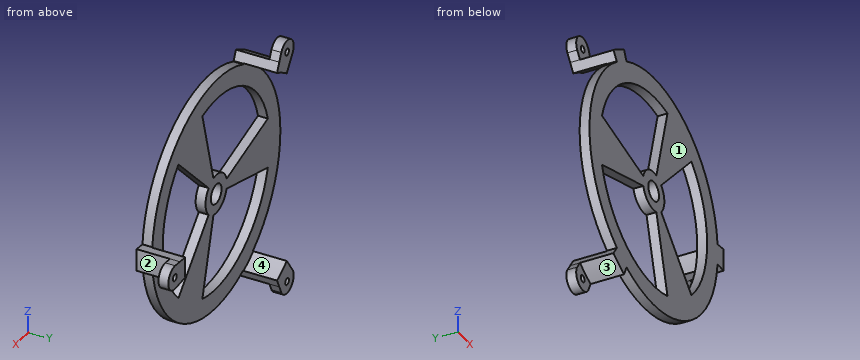
Autodesk Inventor part; units mm, degrees
ref_plane "YZ Plane" through (0, 0, 0) normal (1, 0, 0) x (0, 1, 0)
ref_plane "XZ Plane" through (0, 0, 0) normal (0, 1, 0) x (-1, 0, 0)
ref_plane "XY Plane" through (0, 0, 0) normal (0, 0, 1) x (1, 0, 0)
sketch "Sketch1" plane through (0, 0, 0) normal (0, 1, 0) x (-1, 0, 0)
  line L0 (0, 0) -> (48.2963, -12.941)
  line L1 (0, 0) -> (50, 0) construction
  line L2 (0, 0) -> (48.2963, 12.941)
  line L3 (0, 0) -> (50, 0) construction
  arc A0 (48.2963, -12.941) -> (48.2963, 12.941) centre (0, 0) ccw
  arc A1 (-12.941, 48.2963) -> (-35.3553, 35.3553) centre (0, 0) ccw
  line L4 (0, 0) -> (-12.941, 48.2963)
  line L5 (0, 0) -> (-35.3553, 35.3553)
  arc A2 (-35.3553, -35.3553) -> (-12.941, -48.2963) centre (0, 0) ccw
  line L6 (0, 0) -> (-35.3553, -35.3553)
  line L7 (0, 0) -> (-12.941, -48.2963)
  circle A3 centre (0, 0) radius 5
  circle A4 centre (0, 0) radius 10
  line L8 (0, 0) -> (34.7014, -49.5587)
  line L9 (0, 0) -> (60.5, 0) construction
  line L10 (0, 0) -> (25.5684, -54.8316)
  line L11 (0, 0) -> (60.5, 0) construction
  line L12 (25.5684, -54.8316) -> (27.6815, -59.3632)
  line L13 (34.7014, -49.5587) -> (37.5693, -53.6545)
  arc A5 (27.6815, -59.3632) -> (37.5693, -53.6545) centre (0, 0) ccw
  circle A6 centre (0, 0) radius 50
  circle A7 centre (0, 0) radius 60
  line L14 (0, 0) -> (25.5684, 54.8316)
  line L15 (25.5684, 54.8316) -> (27.6815, 59.3632)
  arc A8 (37.5693, 53.6545) -> (27.6815, 59.3632) centre (0, 0) ccw
  line L16 (0, 0) -> (34.7014, 49.5587)
  line L17 (34.7014, 49.5587) -> (37.5693, 53.6545)
  line L18 (0, 0) -> (-60.2698, -5.2729)
  line L19 (-60.2698, -5.2729) -> (-65.2508, -5.7087)
  arc A9 (-65.2508, 5.7087) -> (-65.2508, -5.7087) centre (0, 0) ccw
  line L20 (0, 0) -> (-60.2698, 5.2729)
  line L21 (-60.2698, 5.2729) -> (-65.2508, 5.7087)
  point P0 (9.6593, -2.5882)
  point P1 (9.6593, 2.5882)
  point P2 (-2.5882, 9.6593)
  point P3 (-7.0711, 7.0711)
  point P4 (-7.0711, -7.0711)
  point P5 (-2.5882, -9.6593)
  point P6 (4.2262, -9.0631)
  point P7 (5.7358, -8.1915)
  point P8 (-35.3553, -35.3553)
  point P9 (-35.3553, 35.3553)
  point P10 (-12.941, 48.2963)
  point P11 (-12.941, -48.2963)
  point P12 (25.3571, -54.3785)
  point P13 (34.4146, -49.1491)
  point P14 (34.4146, 49.1491)
  point P15 (25.3571, 54.3785)
  point P16 (-59.7717, 5.2293)
  point P17 (-59.7717, -5.2293)
  dimension "d0" = 50
  dimension "d1" = 15
  dimension "d2" = 50
  dimension "d3" = 15
  dimension "d4" = 50
  dimension "d7" = 360
  dimension "d9" = 10
  dimension "d10" = 20
  dimension "d11" = 60.5
  dimension "d12" = 55
  dimension "d13" = 60.5
  dimension "d14" = 65
  dimension "d16" = 5
  dimension "d17" = 5
  dimension "d18" = 65.5
  dimension "d25" = 100
  dimension "d26" = 120
  dimension "d29" = 360
extrude "Extrusion2" add sketch "Sketch1" along normal blind 5 contours A3 L2 A4 L0 | L0 A4 L8 A3 | A3 L16 A4 L2 | A3 L5 A4 L4 | L4 A4 L14 A3 | A3 L20 A4 L5 | A3 L7 A4 L6 | L6 A4 L18 A3 | A3 L10 A4 L7 | L8 A4 L10 A3 | L14 A4 L16 A3 | L18 A4 L20 A3 | A4 L2 A0 L0 | A4 L5 A1 L4 | A4 L7 A2 L6 | A0 A6 L16 A7 L8 | A1 A6 L20 A7 L14 | A2 A6 L10 A7 L18 | L8 A7 L10 A6 | L14 A7 L16 A6 | L18 A7 L20 A6 | L8 L13 A5 L12 L10 A7 | L14 L15 A8 L17 L16 A7 | L18 L19 A9 L21 L20 A7
sketch "Sketch3" plane through (0, 5, 0) normal (0, 1, 0) x (1, 0, 0)
  circle A0 centre (0, 0) radius 5
  arc A1 (65.2508, -5.7087) -> (65.2508, 5.7087) centre (0, 0) ccw
  arc A2 (65.2508, -5.7087) -> (65.2508, 5.7087) centre (0, 0) ccw
  line L0 (65.2508, 5.7087) -> (60.2698, 5.2729)
  line L1 (65.2508, 5.7087) -> (59.7717, 5.2293)
  line L2 (65.2508, -5.7087) -> (60.2698, -5.2729)
  line L3 (59.7717, -5.2293) -> (65.2508, -5.7087)
  arc A3 (60.2698, -5.2729) -> (60.2698, 5.2729) centre (0, 0) ccw
  arc A4 (-27.6815, 59.3632) -> (-37.5693, 53.6545) centre (0, 0) ccw
  line L4 (-37.5693, 53.6545) -> (-34.7014, 49.5587)
  arc A5 (-25.5684, 54.8316) -> (-34.7014, 49.5587) centre (0, 0) ccw
  line L5 (-27.6815, 59.3632) -> (-25.5684, 54.8316)
  arc A6 (-37.5693, -53.6545) -> (-27.6815, -59.3632) centre (0, 0) ccw
  line L6 (-27.6815, -59.3632) -> (-25.5684, -54.8316)
  arc A7 (-34.7014, -49.5587) -> (-25.5684, -54.8316) centre (0, 0) ccw
  line L7 (-37.5693, -53.6545) -> (-34.7014, -49.5587)
  dimension "d40" = 5
  dimension "d41" = 5
  dimension "d42" = 60.5
  dimension "d45" = 360
extrude "Extrusion3" add sketch "Sketch3" along normal blind 17 contours L2 A3 L0 A1 | L5 A5 L4 A4 | L7 A7 L6 A6
sketch "Sketch4" plane through (0, 22, 0) normal (0, 1, 0) x (1, 0, 0)
  arc A0 (-27.6815, 59.3632) -> (-37.5693, 53.6545) centre (0, 0) ccw
  arc A1 (-27.6815, 59.3632) -> (-37.5693, 53.6545) centre (0, 0) ccw
  line L0 (-27.6815, 59.3632) -> (-29.5833, 63.4415)
  line L1 (-27.6815, 59.3632) -> (-23.1815, 59.3632) construction
  line L2 (-37.5693, 53.6545) -> (-40.1504, 57.3406)
  line L3 (-37.5693, 53.6545) -> (-33.0693, 53.6545) construction
  circle A2 centre (-35, 60.6218) radius 1.75
  arc A3 (-29.5833, 63.4415) -> (-40.1504, 57.3406) centre (-35, 60.6218) ccw
  arc A4 (-40.1504, -57.3406) -> (-29.5833, -63.4415) centre (-35, -60.6218) ccw
  circle A5 centre (-35, -60.6218) radius 1.75
  line L4 (-37.5693, -53.6545) -> (-40.1504, -57.3406)
  line L5 (-27.6815, -59.3632) -> (-29.5833, -63.4415)
  arc A6 (-37.5693, -53.6545) -> (-27.6815, -59.3632) centre (0, 0) ccw
  arc A7 (69.7336, -6.1009) -> (69.7336, 6.1009) centre (70, 0) ccw
  circle A8 centre (70, 0) radius 1.75
  line L6 (65.2508, -5.7087) -> (69.7336, -6.1009)
  line L7 (65.2508, 5.7087) -> (69.7336, 6.1009)
  arc A9 (65.2508, -5.7087) -> (65.2508, 5.7087) centre (0, 0) ccw
  point P0 (0, 0)
  dimension "d50" = 4.5
  dimension "d51" = 115
  dimension "d52" = 4.5
  dimension "d53" = 125
  dimension "d63" = 3.5
  dimension "d66" = 360
  dimension "d70" = 70
extrude "Extrusion5" add sketch "Sketch4" against normal blind 5
properties part number "MechSwitch_DielecTop"
Check sheet for the modelled part. Datum: model origin and axes. Units: mm. Face numbers are marked on the shaded views. Give positions to 0.01 mm unless a question says otherwise; leave off trailing zeros. Write each loop counter-clockwise with the first axis right and the second up, starting at its lowest first coordinate (ties: lowest second). Pieces come first, ordered by that corner, then holes. Notation, with made-up numbers: (-24, -8.5) -> (17, -8.5) arc R25 ccw to (17, 20.5) -> close; hole circle Ø2 at (51.5, 72.25). An arc over 180 degrees is marked (long way). Use CSV: the item, a comma, the result in double quotes. Start each with the question number.
Q1. Depth check by flat-ended pin: P1, Ø5.5, axis at x = 70.5, z = 1.5, coming from the -Y side; P2, Ø4, axis at y = 4.5, z = 32.5, coming from the +X side; P3, Ø3, axis at y = 12.5, z = -2, coming from the -X side; P4, Ø4.5, axis at x = 70, z = 0, coming from the +Y side. Enter the tip coordinate at first touch or a pass-through.
Q2. Release check for a two-part mould opening along Z. For the marked faces 1, 2, 3 and 4 record: +Z half, -Z half, draft (parallel to the pull), parting line (faces both ways), or undercut.
Q3. Cross-section at B-B on y = 14.25. Enter the section's corners in (x, z), and give its area (3 significant figures).
Q4. Cross-section at D-D on x = 45. Enter the section's corners in (y, z), and give its area (3 significant figures).
Q5. Cross-section at C-C on z = 0. Enter the section's corners in (x, y).
Q6. Scan lines: line 1 along Z through (x, y) = (0, 3.4); line 2 along Z through (x, y) = (-35, 19.55); line 3 along Z through (x, y) = (70, 20.4). Record each from-to range of solid material in increasing order.
Q7. Cross-section at A-A on x = 0. Enter the section's corners in (y, z).
Working result:
1,P1,"stops at y = 17"
1,P2,"stops at x = 51.67"
1,P3,"stops at x = 60.4"
1,P4,"stops at y = 22"
2,face 1,"draft"
2,face 2,"parting line"
2,face 3,"-Z half"
2,face 4,"undercut"
3,outline,"(-37.57, -53.65) arc R65.5 ccw to (-27.68, -59.36) -> (-25.57, -54.83) arc R60.5 cw to (-34.7, -49.56) -> close; (-37.57, 53.65) -> (-34.7, 49.56) arc R60.5 cw to (-25.57, 54.83) -> (-27.68, 59.36) arc R65.5 ccw to start; (60.27, -5.27) -> (65.25, -5.71) arc R65.5 ccw to (65.25, 5.71) -> (60.27, 5.27) arc R60.5 cw to start"
3,area,"165 mm^2"
4,outline,"(0, -39.69) -> (5, -39.69) -> (5, -21.79) -> (0, -21.79) -> close; (0, 21.79) -> (5, 21.79) -> (5, 39.69) -> (0, 39.69) -> close"
4,area,"179 mm^2"
5,outline,"(-60, 0) -> (-5, 0) -> (-5, 5) -> (-60, 5) -> close; (5, 0) -> (10, 0) -> (10, 5) -> (5, 5) -> close; (50, 0) -> (65.5, 0) -> (65.5, 17) -> (68.25, 17) -> (68.25, 22) -> (60.5, 22) -> (60.5, 5) -> (50, 5) -> close; (71.75, 17) -> (76.11, 17) -> (76.11, 22) -> (71.75, 22) -> close"
6,line 1,"z = -60 to -50, -10 to -5, 5 to 10, 50 to 60"
6,line 2,"z = -66.73 to -62.37, -58.87 to -49.99, 49.99 to 58.87, 62.37 to 66.73"
6,line 3,"z = -6.11 to -1.75, 1.75 to 6.11"
7,outline,"(0, -60) -> (5, -60) -> (5, -50) -> (0, -50) -> close; (0, -10) -> (5, -10) -> (5, -5) -> (0, -5) -> close; (0, 5) -> (5, 5) -> (5, 10) -> (0, 10) -> close; (0, 50) -> (5, 50) -> (5, 60) -> (0, 60) -> close"
